Design review of the part shown in the three views and the two pictorial views. Dimensions are in mm from the part's minimum x, y and z. A direction names the side the tool comes from. Give positions to 0.01 mm unless a question says otherwise; leave off trailing zeros. Order: outer loops, then holes, each group sorted by start corner. A loop starts at its lowest first (then second) coordinate and runs counter-clockwise, first axis right, second up.
Item 1: For probe 1 along Z at (x, y) = (25, 7); probe 2 along Z at (x, y) = (150, 30); probe 3 along Y at (x, z) = (23.5, 41), list the stretches that pass through material, from the lowest coordinate up.
Item 2: The part is to be moulded in two halves that separate along Z. For the marked faces 1, 2, 3 and 4, say which applies: released by +Z, released by -Z, zero draft, split by the parting line, or undercut.
Item 3: For P1, Ø1, axis at x = 150.5, y = 31, coming from the +Z side; P2, Ø5, axis at y = 14, z = 33, coming from the -X side; P3, Ø6, axis at x = 97, z = 15, coming from the +Y side, all flat-tipped, find the tip position at first contact; note any pin that passes through.
Item 4: Machinability: for the marked faces 5 and 6, which of the approach directions +Z, -Z, +X, -X, +Y, -Y give a long, thin tool a straight path to every point of the face, cutting with its end or side? Answer none if there is none.
Item 5: Consider section D-D (y = 36). Give the boundary of the cut face in (x, z).
Item 6: Consider section C-C (x = 25). Give the boundary of the cut face in (y, z).
Item 7: Consider section B-B (x = 150). Give the boundary of the cut face in (y, z), plus the area to 3 significant figures.
Item 8: Consider section A-A (z = 25). Give the boundary of the cut face in (x, y) (3 decimals).
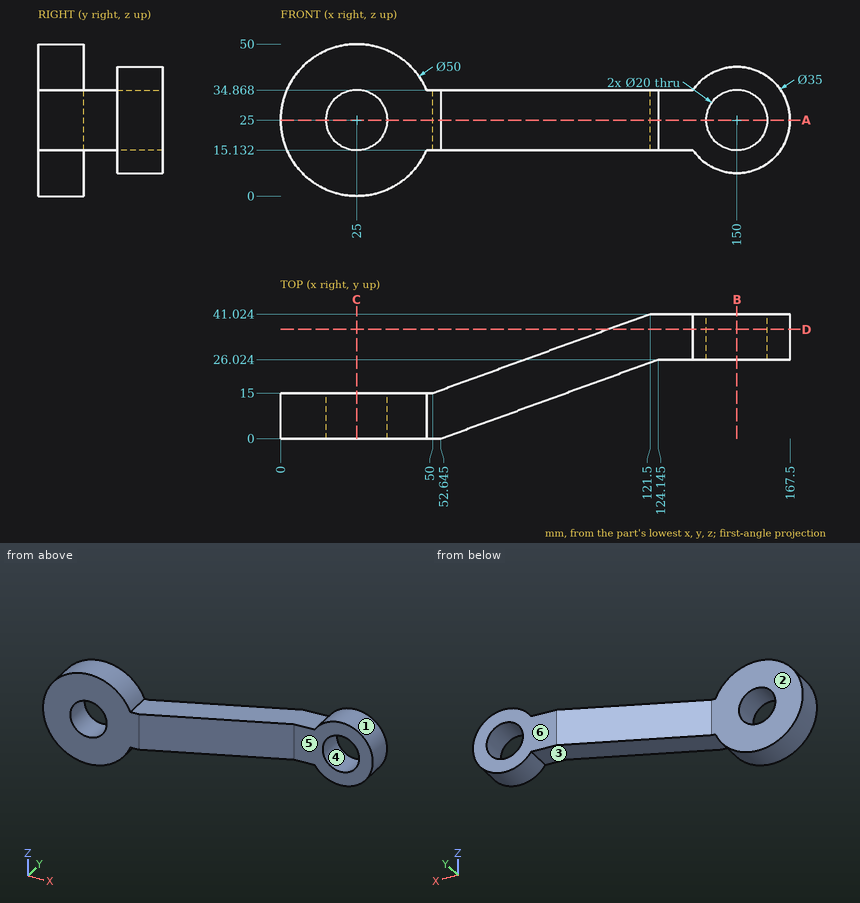
Resolved:
1. probe 1: z = 0 to 15, 35 to 50
1. probe 2: z = 7.5 to 15, 35 to 42.5
1. probe 3: y = 0 to 15
2. face 1: split by the parting line
2. face 2: zero draft
2. face 3: released by -Z
2. face 4: undercut
3. P1: stops at z = 42.5
3. P2: stops at x = 0.61
3. P3: stops at y = 33.2
4. face 5: +Z, -Z, +X, -Y
4. face 6: +Z, -Z, +X, -X, +Y
5. outline: (107.7, 15.13) - (135.55, 15.13) arc R17.5 ccw (long way) to (135.55, 34.87) - (107.7, 34.87) - close; hole circle Ø20 at (150, 25)
6. outline: (0, 0) - (15, 0) - (15, 15) - (0, 15) - close; (0, 35) - (15, 35) - (15, 50) - (0, 50) - close
7. outline: (26.02, 7.5) - (41.02, 7.5) - (41.02, 15) - (26.02, 15) - close; (26.02, 35) - (41.02, 35) - (41.02, 42.5) - (26.02, 42.5) - close
7. area: 225 mm2
8. outline: (0, 0) - (15, 0) - (15, 15) - (0, 15) - close; (35, 0) - (52.645, 0) - (124.145, 26.024) - (140, 26.024) - (140, 41.024) - (121.5, 41.024) - (50, 15) - (35, 15) - close; (160, 26.024) - (167.5, 26.024) - (167.5, 41.024) - (160, 41.024) - close
